Part model, mm, in its own coordinate system. A direction names the side the tool comes from. Round coordinates to 2 decimals unless told otherwise and drop trailing zeros. Write each loop counter-clockwise with the first axis right and the second up, starting at its lowest first coordinate (ties: lowest second). Pieces come first, ordered by that corner, then holes. Notation, with made-up numbers: M -12,-29 L 29,-29 A23 cw 29,-2 Z; hole C 79,16 d8. An arc over 180 degrees is marked long. Answer as a JSON object with one key per item and string values. Group by question number.
1. Drill centre lines: line 1 (Y direction, x = -2.25, z = -195); line 2 (X direction, y = 24, z = -179); line 3 (Z direction, x = 95, y = 31.5). Where is each one in solid material? Low to high. Write a range as from..to.
2. Band-saw the part on B-B, the plane x = 93.5. Write the cut outline in (y, z), plus the area to 3 significant figures.
3. Band-saw the part on A-A, the plane z = -328.5. Write the cut outline in (x, y).
4. Drop flat-ended pins along their axis: pin 1 (2 mm diameter, centred on y = 23.5, z = -205, fed in from -X); pin 2 (2 mm diameter, centred on x = 142.5, y = 22, fed in from +Z). Give the stop position or say it passes through.
5. Which spindle directions (+Z, -Z, +X, -X, +Y, -Y) get a long thin tool onto all of the face, cutting with end or side? Do faces 4 (the face through (-4, 17, -202)), 5 (the face through (13.944, 17.255, -14.34)). Say none if no direction does.
6. Two-plate mould, pull along Z, no slides. Class faces 1 (the face through (156.49, 17.26, -11.12)), 2 (the face through (-1, 35, -201)), 3 (the face through (168, 17, -198)): +Z half, -Z half, draft (parallel to the pull), parting line (faces both ways), or undercut.
from build123d import *

# Parameters (mm, degrees)
Y_KSEKLIK_EKSTR_ZYON1_DEPTH = 35
KES_EKSTR_ZYON1_DEPTH       = 269
IZIM3_R                     = 2
IZIM3_R_2                   = 1.25
KES_EKSTR_ZYON2_DEPTH       = 10
IZIM4_R                     = 2
IZIM4_R_2                   = 1.25
KES_EKSTR_ZYON3_DEPTH       = 10
IZIM5_R                     = 1.25
IZIM5_R_2                   = 2
KES_EKSTR_ZYON4_DEPTH       = 77
IZIM6_R                     = 1.25
IZIM6_R_2                   = 2
KES_EKSTR_ZYON5_DEPTH       = 77
IZIM7_R                     = 2
IZIM7_R_2                   = 1.25
KES_EKSTR_ZYON6_DEPTH       = 382
IZIM8_R                     = 2
IZIM8_R_2                   = 1.25
Y_KSEKLIK_EKSTR_ZYON3_DEPTH = 4
Y_KSEKLIK_EKSTR_ZYON4_START = -4
IZIM9_R                     = 2
IZIM9_R_2                   = 1.25
Y_KSEKLIK_EKSTR_ZYON4_DEPTH = 4
IZIM10_R                    = 2
IZIM10_R_2                  = 1.25
KES_EKSTR_ZYON8_DEPTH       = 228


with BuildPart() as part:
    # Çizim1 → Yükseklik-Ekstrüzyon1 (new body)
    with BuildSketch(Plane(origin=(0, 0, 0), x_dir=(1, 0, 0), z_dir=(0, 1, 0))):
        with BuildLine():
            Line((142.544155877, -2.828427125), (170.828427125, 25.455844123))
            ThreePointArc((170.828427125, 25.455844123), (171.69551813, 26.753537518), (172, 28.284271247))
            Line((172, 28.284271247), (172, 371.715728753))
            ThreePointArc((172, 371.715728753), (171.69551813, 373.246462482), (170.828427125, 374.544155877))
            Line((170.828427125, 374.544155877), (142.544155877, 402.828427125))
            ThreePointArc((142.544155877, 402.828427125), (141.246462482, 403.69551813), (139.715728753, 404))
            Line((139.715728753, 404), (28.284271247, 404))
            ThreePointArc((28.284271247, 404), (26.753537518, 403.69551813), (25.455844123, 402.828427125))
            Line((25.455844123, 402.828427125), (-2.828427125, 374.544155877))
            ThreePointArc((-2.828427125, 374.544155877), (-3.69551813, 373.246462482), (-4, 371.715728753))
            Line((-4, 371.715728753), (-4, 28.284271247))
            ThreePointArc((-4, 28.284271247), (-3.69551813, 26.753537518), (-2.828427125, 25.455844123))
            Line((-2.828427125, 25.455844123), (25.455844123, -2.828427125))
            ThreePointArc((25.455844123, -2.828427125), (26.753537518, -3.69551813), (28.284271247, -4))
            Line((28.284271247, -4), (139.715728753, -4))
            ThreePointArc((139.715728753, -4), (141.246462482, -3.69551813), (142.544155877, -2.828427125))
        make_face()
        Polygon((28.284271247, 0), (139.715728753, 0), (168, 28.284271247), (168, 371.715728753), (139.715728753, 400), (28.284271247, 400), (0, 371.715728753), (0, 28.284271247), align=None, mode=Mode.SUBTRACT)
    extrude(amount=Y_KSEKLIK_EKSTR_ZYON1_DEPTH)

    # Çizim2 → Kes-Ekstrüzyon1 (cut)
    with BuildSketch(Plane(origin=(172, 0, 0), x_dir=(0, 0, -1), z_dir=(1, 0, 0))):
        with BuildLine():
            ThreePointArc((275.468296909, 17.5), (275.456881004, 17.761467228), (275.422720168, 18.020944533))
            Line((275.422720168, 18.020944533), (272.468296909, 17.5))
            Line((272.468296909, 17.5), (275.422720168, 16.979055467))
            ThreePointArc((275.422720168, 16.979055467), (275.456881004, 17.238532772), (275.468296909, 17.5))
        make_face()
        with BuildLine():
            Line((272.468296909, 17.5), (275.422720168, 18.020944533))
            ThreePointArc((275.422720168, 18.020944533), (269.468296909, 17.5), (275.422720168, 16.979055467))
            Line((275.422720168, 16.979055467), (272.468296909, 17.5))
        make_face()
    extrude(amount=-KES_EKSTR_ZYON1_DEPTH, mode=Mode.SUBTRACT)

    # Çizim3 → Kes-Ekstrüzyon2 (cut)
    with BuildSketch(Plane(origin=(272.686291501, 0, -272.686291501), x_dir=(-0.7071067811865404, 0, -0.7071067811865547), z_dir=(0.7071067811865547, 0, -0.7071067811865404))):
        with Locations((176.048773235, 17.5)):
            Circle(IZIM3_R)
        with Locations((164.048773235, 8.5)):
            Circle(IZIM3_R)
        with Locations((164.048773235, 26.5)):
            Circle(IZIM3_R)
        with Locations((152.048773235, 17.5)):
            Circle(IZIM3_R)
        with Locations((158.048773235, 22.5)):
            Circle(IZIM3_R_2)
        with Locations((170.048773235, 22.442626722)):
            Circle(IZIM3_R_2)
        with Locations((158.048773235, 12.5)):
            Circle(IZIM3_R_2)
        with Locations((170.048773235, 12.557373278)):
            Circle(IZIM3_R_2)
    extrude(amount=-KES_EKSTR_ZYON2_DEPTH, mode=Mode.SUBTRACT)

    # Çizim4 → Kes-Ekstrüzyon3 (cut)
    with BuildSketch(Plane(origin=(-188.686291501, 0, -188.686291501), x_dir=(-0.707106781186543, 0, 0.707106781186552), z_dir=(-0.707106781186552, 0, -0.707106781186543))):
        with Locations((-270.842712475, 17.5)):
            Circle(IZIM4_R)
        with Locations((-282.842712475, 26.5)):
            Circle(IZIM4_R)
        with Locations((-282.773588044, 8.5)):
            Circle(IZIM4_R)
        with Locations((-294.842712475, 17.5)):
            Circle(IZIM4_R)
        with Locations((-288.842712475, 22.5)):
            Circle(IZIM4_R_2)
        with Locations((-276.842712475, 22.5)):
            Circle(IZIM4_R_2)
        with Locations((-288.842712475, 12.5)):
            Circle(IZIM4_R_2)
        with Locations((-276.842712475, 12.5)):
            Circle(IZIM4_R_2)
    extrude(amount=-KES_EKSTR_ZYON3_DEPTH, mode=Mode.SUBTRACT)

    # Çizim5 → Kes-Ekstrüzyon4 (cut)
    with BuildSketch(Plane(origin=(11.313708499, 0, -11.313708499), x_dir=(0.7071067811865513, 0, 0.7071067811865438), z_dir=(-0.7071067811865438, 0, 0.7071067811865513))):
        with Locations((6, 23.146313605)):
            Circle(IZIM5_R)
        with Locations((-6, 23.146313605)):
            Circle(IZIM5_R)
        with Locations((0, 27.146313605)):
            Circle(IZIM5_R_2)
        with Locations((0, 8.5)):
            Circle(IZIM5_R_2)
        with Locations((6, 12.5)):
            Circle(IZIM5_R)
        with Locations((-6, 12.5)):
            Circle(IZIM5_R)
        with Locations((10.212993677, 17.5)):
            Circle(IZIM5_R_2)
        with Locations((-11.245301358, 17.5)):
            Circle(IZIM5_R_2)
    extrude(amount=-KES_EKSTR_ZYON4_DEPTH, mode=Mode.SUBTRACT)

    # Çizim6 → Kes-Ekstrüzyon5 (cut)
    with BuildSketch(Plane(origin=(72.686291501, 0, 72.686291501), x_dir=(0.7071067811865476, 0, -0.7071067811865476), z_dir=(0.7071067811865476, 0, 0.7071067811865476))):
        with Locations((124.793939239, 12.5)):
            Circle(IZIM6_R)
        with Locations((112.793939239, 12.5)):
            Circle(IZIM6_R)
        with Locations((112.793939239, 22.5)):
            Circle(IZIM6_R)
        with Locations((118.793939239, 26.5)):
            Circle(IZIM6_R_2)
        with Locations((124.793939239, 22.5)):
            Circle(IZIM6_R)
        with Locations((130.793939239, 17.5)):
            Circle(IZIM6_R_2)
        with Locations((106.793939239, 17.5)):
            Circle(IZIM6_R_2)
        with Locations((118.793939239, 8.5)):
            Circle(IZIM6_R_2)
    extrude(amount=-KES_EKSTR_ZYON5_DEPTH, mode=Mode.SUBTRACT)

    # Çizim7 → Kes-Ekstrüzyon6 (cut)
    with BuildSketch(Plane(origin=(172, 0, 0), x_dir=(0, 0, -1), z_dir=(1, 0, 0))):
        with Locations((200, 26.5)):
            Circle(IZIM7_R)
        with Locations((194, 22.5)):
            Circle(IZIM7_R_2)
        with Locations((206, 22.5)):
            Circle(IZIM7_R_2)
        with Locations((194, 12.5)):
            Circle(IZIM7_R_2)
        with Locations((206, 12.5)):
            Circle(IZIM7_R_2)
        with Locations((200, 8.5)):
            Circle(IZIM7_R)
        with Locations((188, 17.5)):
            Circle(IZIM7_R)
        with Locations((212, 17.5)):
            Circle(IZIM7_R)
    extrude(amount=-KES_EKSTR_ZYON6_DEPTH, mode=Mode.SUBTRACT)

    # Çizim8 → Yükseklik-Ekstrüzyon3 (add)
    with BuildSketch(Plane(origin=(172, 0, 0), x_dir=(0, 0, -1), z_dir=(1, 0, 0))):
        with Locations((200, 26.5)):
            Circle(IZIM8_R)
        with Locations((206, 22.5)):
            Circle(IZIM8_R_2)
        with Locations((194, 22.5)):
            Circle(IZIM8_R_2)
        with Locations((188, 17.5)):
            Circle(IZIM8_R)
        with Locations((194, 12.5)):
            Circle(IZIM8_R_2)
        with Locations((200, 8.5)):
            Circle(IZIM8_R)
        with Locations((206, 12.5)):
            Circle(IZIM8_R_2)
        with Locations((212, 17.5)):
            Circle(IZIM8_R)
    extrude(amount=-Y_KSEKLIK_EKSTR_ZYON3_DEPTH)

    # Çizim9 → Yükseklik-Ekstrüzyon4 (add)
    with BuildSketch(Plane.ZY.offset(4).offset(Y_KSEKLIK_EKSTR_ZYON4_START)):
        with Locations((-200, 26.5)):
            Circle(IZIM9_R)
        with Locations((-194, 22.5)):
            Circle(IZIM9_R_2)
        with Locations((-206, 22.5)):
            Circle(IZIM9_R_2)
        with Locations((-212, 17.5)):
            Circle(IZIM9_R)
        with Locations((-206, 12.5)):
            Circle(IZIM9_R_2)
        with Locations((-200, 8.5)):
            Circle(IZIM9_R)
        with Locations((-194, 12.5)):
            Circle(IZIM9_R_2)
        with Locations((-188, 17.5)):
            Circle(IZIM9_R)
    extrude(amount=Y_KSEKLIK_EKSTR_ZYON4_DEPTH)

    # Çizim10 → Kes-Ekstrüzyon8 (cut)
    with BuildSketch(Plane.ZY.offset(4)):
        with Locations((-200, 29.5)):
            Circle(IZIM10_R)
        with Locations((-209, 17.5)):
            Circle(IZIM10_R)
        with Locations((-191, 17.5)):
            Circle(IZIM10_R)
        with Locations((-200, 5.5)):
            Circle(IZIM10_R)
        with Locations((-205, 23.5)):
            Circle(IZIM10_R_2)
        with Locations((-195, 23.5)):
            Circle(IZIM10_R_2)
        with Locations((-205, 11.5)):
            Circle(IZIM10_R_2)
        with Locations((-195, 11.5)):
            Circle(IZIM10_R_2)
    extrude(amount=-KES_EKSTR_ZYON8_DEPTH, mode=Mode.SUBTRACT)


solid = part.part
Worked answers:
{
 "1": {"line 1": "y = 0..10.25, 12.75..22.25, 24.75..35", "line 2": "x = -4..0, 168..172", "line 3": "z = -404..-400, 0..4"},
 "2": {"outline": "M 0,-404 L 35,-404 L 35,-400 L 0,-400 Z; M 0,0 L 35,0 L 35,4 L 0,4 Z", "area": "280 mm^2"},
 "3": {"outline": "M -4,0 L 0,0 L 0,35 L -4,35 Z; M 168,0 L 172,0 L 172,35 L 168,35 Z"},
 "4": {"pin 1": "passes through", "pin 2": "stops at z = 3.58"},
 "5": {"face 4": "+Z, -Z, -X, +Y, -Y", "face 5": "+Y, -Y"},
 "6": {"face 1": "+Z half", "face 2": "draft", "face 3": "undercut"}
}
